```python
from build123d import *

# Parameters (mm, degrees)
SKETCH1_R           = 200
BOSS_EXTRUDE1_DEPTH = 2
SKETCH2_R           = 2
CUT_EXTRUDE1_DEPTH  = 13
CIRPATTERN1_COUNT   = 4
SKETCH5_R           = 7.5
CUT_EXTRUDE3_DEPTH  = 2
SKETCH7_R           = 2
CUT_EXTRUDE4_DEPTH  = 10
SKETCH8_R           = 1.5
CUT_EXTRUDE5_DEPTH  = 10


with BuildPart() as part:
    # Sketch1 → Boss-Extrude1 (new body)
    with BuildSketch(Plane.XY):
        Circle(SKETCH1_R)
    extrude(amount=BOSS_EXTRUDE1_DEPTH)

    # Sketch2 → Cut-Extrude1 (cut)
    with BuildSketch(Plane(origin=(0, 0, 0), x_dir=(-1, 0, 0), z_dir=(0, 0, -1))):
        with Locations((11.5, 180)):
            Circle(SKETCH2_R)
        with Locations(Location((-11.5, 180, 0), (0, 0, 180))):
            Circle(SKETCH2_R)
    cut_extrude1 = extrude(amount=-CUT_EXTRUDE1_DEPTH, mode=Mode.SUBTRACT)

    # CirPattern1: Cut-Extrude1 ×4 about axis
    cirpattern1_axis = Axis((0, 0, 0), (0, 0, 1))
    for i in range(1, CIRPATTERN1_COUNT):
        add(cut_extrude1.rotate(cirpattern1_axis, i * 360 / CIRPATTERN1_COUNT), mode=Mode.SUBTRACT)

    # Sketch5 → Cut-Extrude3 (cut)
    with BuildSketch(Plane(origin=(0, 0, 0), x_dir=(-1, 0, 0), z_dir=(0, 0, -1))):
        with Locations((151.829580255, 0)):
            Circle(SKETCH5_R)
    extrude(amount=-CUT_EXTRUDE3_DEPTH, mode=Mode.SUBTRACT)

    # Sketch7 → Cut-Extrude4 (cut)
    with BuildSketch(Plane(origin=(0, 0, 0), x_dir=(-1, 0, 0), z_dir=(0, 0, -1))):
        with Locations((127.130690154, -92.412874198)):
            Circle(SKETCH7_R)
        with Locations((104.565936539, -110.629127773)):
            Circle(SKETCH7_R)
        with Locations((65.181140017, -61.842574268)):
            Circle(SKETCH7_R)
        with Locations((87.745893632, -43.626320693)):
            Circle(SKETCH7_R)
    extrude(amount=-CUT_EXTRUDE4_DEPTH, mode=Mode.SUBTRACT)

    # Sketch8 → Cut-Extrude5 (cut)
    with BuildSketch(Plane(origin=(0, 0, 0), x_dir=(-1, 0, 0), z_dir=(0, 0, -1))):
        with Locations((-15.432875064, 20.159522992)):
            Circle(SKETCH8_R)
        with Locations((13.948214091, 21.213847451)):
            Circle(SKETCH8_R)
        with Locations((-13.216642017, -41.60072564)):
            Circle(SKETCH8_R)
        with Locations((16.164447138, -40.546401181)):
            Circle(SKETCH8_R)
    extrude(amount=-CUT_EXTRUDE5_DEPTH, mode=Mode.SUBTRACT)


solid = part.part
```
CAD build for the part. Positions are in the model's coordinates, mm. Round coordinates to 2 decimals unless told otherwise and drop trailing zeros. Order: outer loops, then holes, each group sorted by start corner. A loop starts at its lowest first (then second) coordinate and runs counter-clockwise, first axis right, second up.
Item 1: Saw through at A-A on z = 0.45. State how many separate pieces and enclosed holes the cut face has, then the cut area to 3 significant figures.
Item 2: Mould opens along X. For faces 1 (the face through (190.764, 60.075, 0.986)), 2 (the face through (-144.337, 0.33, 0.986)), 3 (the face through (-3, 3, 0)) say: pulls with the +X half, pulls with the -X half, needs draft (parallel to the pull), parting line crosses it, or undercut.
Item 3: Pin check, flat tips, straight feed: pin 1 (3 mm diameter, centred on x = -11.5, y = -180, fed in from -Z); pin 2 (1 mm diameter, centred on x = 122, z = 1.5, fed in from +Y). Stop position of each tip, or through.
Item 4: Saw through at C-C on x = 130. Write the cut outline in (y, z).
Item 5: Probe line 1 along X through (y, z) = (-11.5, 0.55); line 2 along X through (y, z) = (180, 1.2). List the from-to ranges inside material, lowest first.
Item 6: Saw through at B-B on y = 58. Write the cut outline in (x, z), then the cut area to 3 significant figures.
Reported:
1. separate pieces: 1
1. enclosed holes: 17
1. area: 125,000 mm2
2. face 1: parting line crosses it
2. face 2: undercut
2. face 3: needs draft
3. pin 1: passes through
3. pin 2: stops at y = 158.86
4. outline: (-151.99, 0) - (151.99, 0) - (151.99, 2) - (-151.99, 2) - close
5. line 1: x = -199.67 to -182, -178 to 178, 182 to 199.67
5. line 2: x = -87.18 to -13.5, -9.5 to 9.5, 13.5 to 87.18
6. outline: (-191.41, 0) - (191.41, 0) - (191.41, 2) - (-191.41, 2) - close
6. area: 766 mm2
